```python
from build123d import *

# Parameters (mm, degrees)
F0_W      = 25.4
F0_H      = 127
F1_DEPTH  = 6.35
F2_W      = 12.7
F2_H      = 12.7
F3_DEPTH  = 273.05
F4_W      = 2.54
F4_H      = 6.5340787411
F5_DEPTH  = 25.4
F7_DEPTH  = 5.08
F8_DEPTH  = 25.4
F10_DEPTH = 25.4
F11_R     = 1.27
F12_DEPTH = 25.4


with BuildPart() as f1:
    # F0 (on Top) → F1 (new body)
    with BuildSketch(Plane.XY):
        with Locations((-12.7, 63.5)):
            Rectangle(F0_W, F0_H)
    extrude(amount=F1_DEPTH)

    # F2 (on face) → F3 (join)
    with BuildSketch(Plane.XY.offset(6.35)):
        with Locations((-19.05, 120.65)):
            Rectangle(F2_W, F2_H)
    extrude(amount=F3_DEPTH)

    # F4 (on face) → F5 (join)
    with BuildSketch(Plane.XZ.offset(-114.3)):
        with Locations((-20.32, 276.1329606295)):
            Rectangle(F4_W, F4_H)
    extrude(amount=F5_DEPTH)

    # F6 (on face) → F7 (join)
    with BuildSketch(Plane(origin=(-21.59, 0, 0), x_dir=(0, -1, 0), z_dir=(-1, 0, 0))):
        Polygon((-13.335, 13.97), (-5.715, 13.97), (-111.6269677877, 272.8659212589), (-114.3, 272.8659212589), (-114.3, 263.1782591343), (-114.3, 6.35), (-106.68, 6.35), (-106.68, 13.97), (-106.68, 217.2529995441), (-106.68, 237.5801540886), align=None)
        Polygon((0, 0), (-5.715, 13.97), (-13.335, 13.97), (-106.68, 13.97), (-106.68, 6.35), (-114.3, 6.35), (-114.3, 0), (-96.3151082397, 0), align=None)
    extrude(amount=-F7_DEPTH)

    # F8 (cut): a face of the model
    f8_faces = [f1.faces().sort_by_distance(p)[0] for p in [
        (-20.32, 88.9, 276.1329606295),
    ]]
    extrude(f8_faces, amount=-F8_DEPTH, mode=Mode.SUBTRACT)

    # F9 (on face) → F10 (cut)
    with BuildSketch(Plane.XY.offset(6.35)):
        with BuildLine():
            ThreePointArc((-6.35, 86.2650498748), (-8.5180256121, 87.1630754869), (-7.62, 84.9950498748))
            ThreePointArc((-7.62, 84.9950498748), (-6.7219743879, 85.3670242627), (-6.35, 86.2650498748))
        make_face()
        with BuildLine():
            ThreePointArc((-7.62, 19.2763266307), (-8.5180256121, 17.1083010186), (-6.35, 18.0063266307))
            Line((-6.35, 18.0063266307), (-7.62, 18.0063266307))
            Line((-7.62, 18.0063266307), (-7.62, 19.2763266307))
        make_face()
        with BuildLine():
            Line((-7.62, 18.0063266307), (-6.35, 18.0063266307))
            ThreePointArc((-6.35, 18.0063266307), (-6.7219743879, 18.9043522428), (-7.62, 19.2763266307))
            Line((-7.62, 19.2763266307), (-7.62, 18.0063266307))
        make_face()
    extrude(amount=-F10_DEPTH, mode=Mode.SUBTRACT)

    # F11 (on face) → F12 (cut)
    with BuildSketch(Plane.YZ.offset(-12.7)):
        with BuildLine():
            ThreePointArc((121.92, 266.7), (121.5480256121, 267.5980256121), (120.65, 267.97))
            ThreePointArc((120.65, 267.97), (119.7519743879, 265.8019743879), (121.92, 266.7))
        make_face()
        with Locations((120.65, 231.14)):
            Circle(F11_R)
        with Locations((120.65, 195.58)):
            Circle(F11_R)
        with Locations((120.65, 160.02)):
            Circle(F11_R)
        with Locations((120.65, 124.46)):
            Circle(F11_R)
        with Locations((120.65, 88.9)):
            Circle(F11_R)
        with Locations((120.65, 53.34)):
            Circle(F11_R)
        with Locations((120.65, 17.78)):
            Circle(F11_R)
    extrude(amount=-F12_DEPTH, mode=Mode.SUBTRACT)


solid = f1.part
```
Build history of the part. All positions in model axes, mm. A direction names the side the tool comes from. Give positions to 0.01 mm unless a question says otherwise; leave off trailing zeros. Loops run counter-clockwise (first coordinate to the right, second up) from the corner with the lowest first, then second, coordinate; pieces in that order, holes last. Notation, with made-up numbers: (9.25, 72) -> (17.25, 72) arc R10 ccw to (17.25, 83) -> close; hole circle Ø1 at (80, 86). An arc over 180 degrees is marked (long way). One line per question, with ' | ' between items. Start each with the question number.
1) 3-axis set-ups, long thin cutter, end or side, ignore diameter. For faces 5 (the flat face through (-12.7, 121, 141)), 6 (the flat face through (-21.59, 55, 120)), 7 (the flat face through (-10, 64, 6.35)), 8 (the flat face through (-16.51, 55, 120)): which of +Z, -Z, +X, -X, +Y, -Y reach the whole face in a straight line?
2) Pin check, flat tips, straight feed: pin 1 (10 mm diameter, centred on x = -5, y = 16.5, fed in from +Z); pin 2 (14 mm diameter, centred on x = -17.5, z = 118.5, fed in from -Y); pin 3 (5.5 mm diameter, centred on x = -18.5, y = 75.5, fed in from +Z). Stop position of each tip, or through.
3) Cut at B-B (z = 140.5). Give the cut face in (x, y), plus the area to 3 significant figures.
4) Two-plate mould, pull along Z, no slides. Class faces 1 (the flat face through (-19, 106.68, 124)), 2 (the flat face through (-13, 64, 0)), 3 (the flat face through (-13, 0, 3)), 4 (the flat face through (-19, 59, 13.97)): released by +Z, released by -Z, zero draft, split by the parting line, or undercut.
5) Cut at A-A (y = 26). Give the cut face in (x, z).
6) Probe L1, parallel to Y at x = -7.62, z = 4; L2, parallel to Y at x = -19.5, z = 160.02; L3, parallel to Y at x = -18, z = 157. List the from-to ranges inside material, lowest first.
Return value:
1) face 5: +Z, +X, +Y, -Y | face 6: +Z, -X, -Y | face 7: +Z, -Y | face 8: +Z, +X, -Y
2) pin 1: z = 6.35 | pin 2: y = 45.61 | pin 3: z = 191.28
3) outline: (-25.4, 114.3) -> (-21.59, 114.3) -> (-21.59, 106.68) -> (-16.51, 106.68) -> (-16.51, 114.3) -> (-12.7, 114.3) -> (-12.7, 127) -> (-25.4, 127) -> close; (-21.59, 57.48) -> (-16.51, 57.48) -> (-16.51, 66.15) -> (-21.59, 66.15) -> close | area: 244 mm^2
4) face 1: undercut | face 2: released by -Z | face 3: zero draft | face 4: undercut
5) outline: (-25.4, 0) -> (0, 0) -> (0, 6.35) -> (-16.51, 6.35) -> (-16.51, 13.97) -> (-21.59, 13.97) -> (-21.59, 6.35) -> (-25.4, 6.35) -> close; (-21.59, 44.31) -> (-16.51, 44.31) -> (-16.51, 63.56) -> (-21.59, 63.56) -> close
6) L1: 0 to 16.74, 19.28 to 85, 87.54 to 127 | L2: 65.46 to 74.3, 106.68 to 119.38, 121.92 to 127 | L3: 64.23 to 73.04, 106.68 to 127
